Can you work these out from the model? Positions are in its coordinate system, mm. Coordinates: 2 decimals unless noted, no trailing zeros. Answer as CSV lines item,"result". Start each with the question number.
```python
from build123d import *

# Parameters (mm, degrees)
F0_R     = 39.6875
F0_R_2   = 0.41275
F0_R_3   = 0.889
F0_R_4   = 2.38125
F1_DEPTH = 3.175


with BuildPart() as f1:
    # F0 (on Front) → F1 (new body)
    with BuildSketch(Plane.XZ):
        Circle(F0_R)
        with Locations((-22.861173, -31.465705)):
            Circle(F0_R_2, mode=Mode.SUBTRACT)
        with Locations((-31.465705, -22.861173)):
            Circle(F0_R_2, mode=Mode.SUBTRACT)
        with Locations((-26.024999, -28.903689)):
            Circle(F0_R_2, mode=Mode.SUBTRACT)
        with Locations((-28.903689, -26.024999)):
            Circle(F0_R_2, mode=Mode.SUBTRACT)
        with Locations((-15.819513, -35.531209)):
            Circle(F0_R_2, mode=Mode.SUBTRACT)
        with Locations((-12.01883, -36.990154)):
            Circle(F0_R_2, mode=Mode.SUBTRACT)
        with Locations((-19.446875, -33.682976)):
            Circle(F0_R_2, mode=Mode.SUBTRACT)
        with Locations((-8.086465, -38.043828)):
            Circle(F0_R_2, mode=Mode.SUBTRACT)
        with Locations((-4.065504, -38.680686)):
            Circle(F0_R_2, mode=Mode.SUBTRACT)
        with Locations((-35.531209, -15.819513)):
            Circle(F0_R_2, mode=Mode.SUBTRACT)
        with Locations((-33.682976, -19.446875)):
            Circle(F0_R_2, mode=Mode.SUBTRACT)
        with Locations((-36.990154, -12.01883)):
            Circle(F0_R_2, mode=Mode.SUBTRACT)
        with Locations((-38.043828, -8.086465)):
            Circle(F0_R_2, mode=Mode.SUBTRACT)
        with Locations((-38.680686, -4.065504)):
            Circle(F0_R_2, mode=Mode.SUBTRACT)
        with BuildLine():
            ThreePointArc((-37.989555, -2.898913), (-37.571111, -1.699143), (-36.406657, -1.190625))
            Line((-36.406657, -1.190625), (-10.759632, -1.190625))
            ThreePointArc((-10.759632, -1.190625), (-9.787491, -1.523096), (-9.222542, -2.38125))
            ThreePointArc((-9.222542, -2.38125), (-6.735192, -6.735192), (-2.38125, -9.222542))
            ThreePointArc((-2.38125, -9.222542), (-1.523096, -9.787491), (-1.190625, -10.759632))
            Line((-1.190625, -10.759632), (-1.190625, -36.406657))
            ThreePointArc((-1.190625, -36.406657), (-1.699143, -37.571111), (-2.898913, -37.989555))
            ThreePointArc((-2.898913, -37.989555), (-26.940768, -26.940768), (-37.989555, -2.898913))
        make_face(mode=Mode.SUBTRACT)
        with Locations((0, -38.89375)):
            Circle(F0_R_2, mode=Mode.SUBTRACT)
        with Locations((4.065504, -38.680686)):
            Circle(F0_R_2, mode=Mode.SUBTRACT)
        with Locations((8.086465, -38.043828)):
            Circle(F0_R_2, mode=Mode.SUBTRACT)
        with Locations((12.01883, -36.990154)):
            Circle(F0_R_2, mode=Mode.SUBTRACT)
        with Locations((15.819513, -35.531209)):
            Circle(F0_R_2, mode=Mode.SUBTRACT)
        with Locations((19.446875, -33.682976)):
            Circle(F0_R_2, mode=Mode.SUBTRACT)
        with Locations((22.861173, -31.465705)):
            Circle(F0_R_2, mode=Mode.SUBTRACT)
        with Locations((26.024999, -28.903689)):
            Circle(F0_R_2, mode=Mode.SUBTRACT)
        with Locations((28.903689, -26.024999)):
            Circle(F0_R_2, mode=Mode.SUBTRACT)
        with Locations((31.465705, -22.861173)):
            Circle(F0_R_2, mode=Mode.SUBTRACT)
        with BuildLine():
            ThreePointArc((2.898913, -37.989555), (1.699143, -37.571111), (1.190625, -36.406657))
            Line((1.190625, -36.406657), (1.190625, -10.759632))
            ThreePointArc((1.190625, -10.759632), (1.523096, -9.787491), (2.38125, -9.222542))
            ThreePointArc((2.38125, -9.222542), (6.735192, -6.735192), (9.222542, -2.38125))
            ThreePointArc((9.222542, -2.38125), (9.787491, -1.523096), (10.759632, -1.190625))
            Line((10.759632, -1.190625), (36.406657, -1.190625))
            ThreePointArc((36.406657, -1.190625), (37.571111, -1.699143), (37.989555, -2.898913))
            ThreePointArc((37.989555, -2.898913), (26.940768, -26.940768), (2.898913, -37.989555))
        make_face(mode=Mode.SUBTRACT)
        with Locations((0, -5.953125)):
            Circle(F0_R_3, mode=Mode.SUBTRACT)
        with Locations((33.682976, -19.446875)):
            Circle(F0_R_2, mode=Mode.SUBTRACT)
        with Locations((35.531209, -15.819513)):
            Circle(F0_R_2, mode=Mode.SUBTRACT)
        with Locations((36.990154, -12.01883)):
            Circle(F0_R_2, mode=Mode.SUBTRACT)
        with Locations((38.043828, -8.086465)):
            Circle(F0_R_2, mode=Mode.SUBTRACT)
        with Locations((38.680686, -4.065504)):
            Circle(F0_R_2, mode=Mode.SUBTRACT)
        with Locations((-38.89375, 0)):
            Circle(F0_R_2, mode=Mode.SUBTRACT)
        with Locations((-38.680686, 4.065504)):
            Circle(F0_R_2, mode=Mode.SUBTRACT)
        with Locations((-38.043828, 8.086465)):
            Circle(F0_R_2, mode=Mode.SUBTRACT)
        with Locations((-36.990154, 12.01883)):
            Circle(F0_R_2, mode=Mode.SUBTRACT)
        with Locations((-35.531209, 15.819513)):
            Circle(F0_R_2, mode=Mode.SUBTRACT)
        with Locations((-33.682976, 19.446875)):
            Circle(F0_R_2, mode=Mode.SUBTRACT)
        with Locations((-5.155557, 2.976563)):
            Circle(F0_R_3, mode=Mode.SUBTRACT)
        with BuildLine():
            ThreePointArc((-37.989555, 2.898913), (-26.940768, 26.940768), (-2.898913, 37.989555))
            ThreePointArc((-2.898913, 37.989555), (-1.699143, 37.571111), (-1.190625, 36.406657))
            Line((-1.190625, 36.406657), (-1.190625, 10.759632))
            ThreePointArc((-1.190625, 10.759632), (-1.523096, 9.787491), (-2.38125, 9.222542))
            ThreePointArc((-2.38125, 9.222542), (-6.735192, 6.735192), (-9.222542, 2.38125))
            ThreePointArc((-9.222542, 2.38125), (-9.787491, 1.523096), (-10.759632, 1.190625))
            Line((-10.759632, 1.190625), (-36.406657, 1.190625))
            ThreePointArc((-36.406657, 1.190625), (-37.571111, 1.699143), (-37.989555, 2.898913))
        make_face(mode=Mode.SUBTRACT)
        with Locations((-31.465705, 22.861173)):
            Circle(F0_R_2, mode=Mode.SUBTRACT)
        with Locations((-28.903689, 26.024999)):
            Circle(F0_R_2, mode=Mode.SUBTRACT)
        with Locations((-26.024999, 28.903689)):
            Circle(F0_R_2, mode=Mode.SUBTRACT)
        with Locations((-22.861173, 31.465705)):
            Circle(F0_R_2, mode=Mode.SUBTRACT)
        with Locations((-19.446875, 33.682976)):
            Circle(F0_R_2, mode=Mode.SUBTRACT)
        with Locations((-15.819513, 35.531209)):
            Circle(F0_R_2, mode=Mode.SUBTRACT)
        with Locations((-12.01883, 36.990154)):
            Circle(F0_R_2, mode=Mode.SUBTRACT)
        with Locations((-8.086465, 38.043828)):
            Circle(F0_R_2, mode=Mode.SUBTRACT)
        with Locations((-4.065504, 38.680686)):
            Circle(F0_R_2, mode=Mode.SUBTRACT)
        Circle(F0_R_4, mode=Mode.SUBTRACT)
        with Locations((5.155557, 2.976562)):
            Circle(F0_R_3, mode=Mode.SUBTRACT)
        with BuildLine():
            Line((1.190625, 10.759632), (1.190625, 36.406657))
            ThreePointArc((1.190625, 36.406657), (1.699143, 37.571111), (2.898913, 37.989555))
            ThreePointArc((2.898913, 37.989555), (26.940768, 26.940768), (37.989555, 2.898913))
            ThreePointArc((37.989555, 2.898913), (37.571111, 1.699143), (36.406657, 1.190625))
            Line((36.406657, 1.190625), (10.759632, 1.190625))
            ThreePointArc((10.759632, 1.190625), (9.787491, 1.523096), (9.222542, 2.38125))
            ThreePointArc((9.222542, 2.38125), (6.735192, 6.735192), (2.38125, 9.222542))
            ThreePointArc((2.38125, 9.222542), (1.523096, 9.787491), (1.190625, 10.759632))
        make_face(mode=Mode.SUBTRACT)
        with Locations((38.89375, 0)):
            Circle(F0_R_2, mode=Mode.SUBTRACT)
        with Locations((38.680686, 4.065504)):
            Circle(F0_R_2, mode=Mode.SUBTRACT)
        with Locations((38.043828, 8.086465)):
            Circle(F0_R_2, mode=Mode.SUBTRACT)
        with Locations((36.990154, 12.01883)):
            Circle(F0_R_2, mode=Mode.SUBTRACT)
        with Locations((33.682976, 19.446875)):
            Circle(F0_R_2, mode=Mode.SUBTRACT)
        with Locations((35.531209, 15.819513)):
            Circle(F0_R_2, mode=Mode.SUBTRACT)
        with Locations((0, 38.89375)):
            Circle(F0_R_2, mode=Mode.SUBTRACT)
        with Locations((4.065504, 38.680686)):
            Circle(F0_R_2, mode=Mode.SUBTRACT)
        with Locations((8.086465, 38.043828)):
            Circle(F0_R_2, mode=Mode.SUBTRACT)
        with Locations((19.446875, 33.682976)):
            Circle(F0_R_2, mode=Mode.SUBTRACT)
        with Locations((12.01883, 36.990154)):
            Circle(F0_R_2, mode=Mode.SUBTRACT)
        with Locations((15.819513, 35.531209)):
            Circle(F0_R_2, mode=Mode.SUBTRACT)
        with Locations((28.903689, 26.024999)):
            Circle(F0_R_2, mode=Mode.SUBTRACT)
        with Locations((26.024999, 28.903689)):
            Circle(F0_R_2, mode=Mode.SUBTRACT)
        with Locations((31.465705, 22.861173)):
            Circle(F0_R_2, mode=Mode.SUBTRACT)
        with Locations((22.861173, 31.465705)):
            Circle(F0_R_2, mode=Mode.SUBTRACT)
    extrude(amount=F1_DEPTH)


solid = f1.part
```
Q1. For pin 1 (1.6 mm diameter, centred on x = -19.5, y = -1.5, fed in from -Z); pin 2 (1 mm diameter, centred on y = -1.5, z = -27, fed in from +X); pin 3 (1 mm diameter, centred on x = -27.5, y = -2.5, fed in from +Z), each with a flat end and sliding along its axis, tell me the tip position at first contact or that it passes through.
Q2. Imagine slicing it at A-A (y = -2.25). State how many separate pieces and enclosed holes the cut face has, then the cut area to 3 significant figures.
Q3. I need wall thicknesses on L1, parallel to Z at x = 26, y = -2.6; L2, parallel to X at y = -1.55, z = -16; L3, parallel to Z at x = 5.5, y = -1.75. Which ranges of each line are inside material? Lowest first, please.
Q4. If we mould it in two halves opening along X, with no side actions, what happens to faces 1 (the face through (-1.71, -1.57, 37.58)), 2 (the face through (-3, 0, 0))? For each: released by +X, released by -X, zero draft, split by the parting line, or undercut.
Entries:
1,pin 1,"z = -35.01"
1,pin 2,"x = 29.54"
1,pin 3,"z = 29.09"
2,separate pieces,"1"
2,enclosed holes,"68"
2,area,"896 mm2"
3,L1,"-29.98 to -29.32, -28.49 to -27.85, -1.19 to 1.19, 27.85 to 28.49, 29.32 to 29.98"
3,L2,"-36.32 to -35.9, -35.16 to -34.58, -1.19 to 1.19, 34.58 to 35.16, 35.9 to 36.32"
3,L3,"-39.3 to -37.7, -7.78 to 2.16, 3.8 to 7.78, 37.7 to 39.3"
4,face 1,"undercut"
4,face 2,"zero draft"
